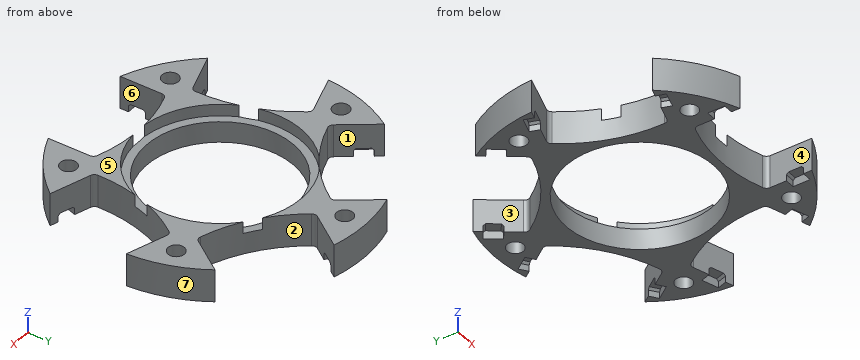
```python
from build123d import *

# Parameters (mm, degrees)
SKETCH1_R                = 28.194
SKETCH1_R_2              = 15.875
SKETCH1_R_3              = 14.2875
BOSS_EXTRUDE1_DEPTH      = 6.35
SKETCH1_3_R              = 15.875
SKETCH1_3_R_2            = 14.2875
CUT_EXTRUDE1_DEPTH       = 2.286
CUT_EXTRUDE5_DEPTH       = 7.35
CIRPATTERN1_COUNT        = 5
CUT_EXTRUDE6_DEPTH       = 1.8796
CIRPATTERN2_COUNT        = 5
CIRPATTERN2_COPY_1_DEPTH = 1.8796
CIRPATTERN2_COPY_2_DEPTH = 1.8796
CIRPATTERN2_COPY_3_DEPTH = 1.8796
CIRPATTERN2_COPY_4_DEPTH = 1.8796
SKETCH4_R                = 1.5875
CUT_EXTRUDE7_DEPTH       = 7.35
CIRPATTERN3_COUNT        = 5


with BuildPart() as part:
    # Sketch1 → Boss-Extrude1 (new body)
    with BuildSketch(Plane.XY):
        Circle(SKETCH1_R)
        Circle(SKETCH1_R_2, mode=Mode.SUBTRACT)
        Circle(SKETCH1_R_2)
        Circle(SKETCH1_R_3, mode=Mode.SUBTRACT)
    extrude(amount=-BOSS_EXTRUDE1_DEPTH)

    # Sketch1_3 → Cut-Extrude1 (cut)
    with BuildSketch(Plane.XY):
        Circle(SKETCH1_3_R)
        Circle(SKETCH1_3_R_2, mode=Mode.SUBTRACT)
    extrude(amount=-CUT_EXTRUDE1_DEPTH, mode=Mode.SUBTRACT)

    # Sketch2 → Cut-Extrude5 (cut, through all)
    with BuildSketch(Plane.XY):
        with BuildLine():
            Line((-10.033, -28.194), (10.033, -28.194))
            Line((10.033, -28.194), (10.033, -18.273516145))
            ThreePointArc((10.033, -18.273516145), (9.84417878, -17.683574397), (9.347899083, -17.312911233))
            ThreePointArc((9.347899083, -17.312911233), (0, -15.748), (-9.347899083, -17.312911233))
            ThreePointArc((-9.347899083, -17.312911233), (-9.84417878, -17.683574397), (-10.033, -18.273516145))
            Line((-10.033, -18.273516145), (-10.033, -28.194))
        make_face()
    cut_extrude5 = extrude(amount=-CUT_EXTRUDE5_DEPTH, mode=Mode.SUBTRACT)

    # CirPattern1: Cut-Extrude5 ×5 about axis
    cirpattern1_axis = Axis((0, 0, 0), (0, 0, 1))
    for i in range(1, CIRPATTERN1_COUNT):
        add(cut_extrude5.rotate(cirpattern1_axis, i * 360 / CIRPATTERN1_COUNT), mode=Mode.SUBTRACT)

    # Sketch3 → Cut-Extrude6 (cut)
    with BuildSketch(Plane(origin=(-10.033, 0, 0), x_dir=(0, 0, -1), z_dir=(1, 0, 0))):
        Polygon((6.35, -21.433544869), (5.15112, -21.433544869), (4.7498, -21.834864869), (4.7498, -24.334224869), (5.15112, -24.735544869), (6.35, -24.735544869), align=None)
    cut_extrude6 = extrude(amount=-CUT_EXTRUDE6_DEPTH, mode=Mode.SUBTRACT)

    # Mirror1: Cut-Extrude6 across plane
    add(cut_extrude6.mirror(Plane(origin=(0, 0, 0), x_dir=(0, 0, 1), z_dir=(1, 0, 0))), mode=Mode.SUBTRACT)

    # CirPattern2: Cut-Extrude6 ×5 about axis
    cirpattern2_axis = Axis((0, 0, 0), (0, 0, 1))
    for i in range(1, CIRPATTERN2_COUNT):
        add(cut_extrude6.rotate(cirpattern2_axis, i * 360 / CIRPATTERN2_COUNT), mode=Mode.SUBTRACT)

    # CirPattern2 copy 1 sketch → CirPattern2 copy 1 (cut)
    with BuildSketch(Plane(origin=(3.100367505, 9.541950028, 0), x_dir=(0, 0, -1), z_dir=(-0.309016994, -0.951056516, 0))):
        Polygon((6.35, 21.433544869), (5.15112, 21.433544869), (4.7498, 21.834864869), (4.7498, 24.334224869), (5.15112, 24.735544869), (6.35, 24.735544869), align=None)
    extrude(amount=-CIRPATTERN2_COPY_1_DEPTH, mode=Mode.SUBTRACT)

    # CirPattern2 copy 2 sketch → CirPattern2 copy 2 (cut)
    with BuildSketch(Plane(origin=(-8.116867505, 5.897249436, 0), x_dir=(0, 0, -1), z_dir=(0.809016994, -0.587785252, 0))):
        Polygon((6.35, 21.433544869), (5.15112, 21.433544869), (4.7498, 21.834864869), (4.7498, 24.334224869), (5.15112, 24.735544869), (6.35, 24.735544869), align=None)
    extrude(amount=-CIRPATTERN2_COPY_2_DEPTH, mode=Mode.SUBTRACT)

    # CirPattern2 copy 3 sketch → CirPattern2 copy 3 (cut)
    with BuildSketch(Plane(origin=(-8.116867505, -5.897249436, 0), x_dir=(0, 0, -1), z_dir=(0.809016994, 0.587785252, 0))):
        Polygon((6.35, 21.433544869), (5.15112, 21.433544869), (4.7498, 21.834864869), (4.7498, 24.334224869), (5.15112, 24.735544869), (6.35, 24.735544869), align=None)
    extrude(amount=-CIRPATTERN2_COPY_3_DEPTH, mode=Mode.SUBTRACT)

    # CirPattern2 copy 4 sketch → CirPattern2 copy 4 (cut)
    with BuildSketch(Plane(origin=(3.100367505, -9.541950028, 0), x_dir=(0, 0, -1), z_dir=(-0.309016994, 0.951056516, 0))):
        Polygon((6.35, 21.433544869), (5.15112, 21.433544869), (4.7498, 21.834864869), (4.7498, 24.334224869), (5.15112, 24.735544869), (6.35, 24.735544869), align=None)
    extrude(amount=-CIRPATTERN2_COPY_4_DEPTH, mode=Mode.SUBTRACT)

    # Sketch4 → Cut-Extrude7 (cut, through all)
    with BuildSketch(Plane(origin=(0, 0, -6.35), x_dir=(-1, 0, 0), z_dir=(0, 0, -1))):
        with Locations((-14.191068427, -19.532330016)):
            Circle(SKETCH4_R)
    cut_extrude7 = extrude(amount=-CUT_EXTRUDE7_DEPTH, mode=Mode.SUBTRACT)

    # CirPattern3: Cut-Extrude7 ×5 about axis
    cirpattern3_axis = Axis((0, 0, 0), (0, 0, 1))
    for i in range(1, CIRPATTERN3_COUNT):
        add(cut_extrude7.rotate(cirpattern3_axis, i * 360 / CIRPATTERN3_COUNT), mode=Mode.SUBTRACT)


solid = part.part
```
CAD build for the part. Positions are in the model's coordinates, mm. Face numbers are marked on the shaded views. A direction names the side the tool comes from. Round coordinates to 2 decimals unless told otherwise and drop trailing zeros. Loops run counter-clockwise (first coordinate to the right, second up) from the corner with the lowest first, then second, coordinate; pieces in that order, holes last. Notation, with made-up numbers: M 40.25,65.5 L 57.25,65.5 A30 cw 57.25,99.5 Z; hole C 2.25,13 d11. An arc over 180 degrees is marked long. Return JSON: item names as keys, results as strings. Group by question number.
(1) Wall check: probe 1 along Y at (x, z) = (0, -5); probe 2 along X at (y, z) = (12.5, -3.5). Give the ranges that are in metal, low to high. Write a range as [from, to].
(2) Drop flat-ended pins along their axis: P1, Ø2.5, axis at x = -14.19, y = -19.53, coming from the +Z side; P2, Ø2, axis at x = -25.5, y = 2.5, coming from the -Z side (3 decimals); P3, Ø1.3, axis at x = 18.5, y = -17.5, coming from the -Z side; P4, Ø1, axis at x = -11, z = -5.5, coming from the -Y side. Give the stop position or say it passes through.
(3) Saw through at A-A, the plane x = 0. Give the number of separate pieces and of enclosed holes in the cut face, and give its area (3 significant figures).
(4) Tool access for the marked faces 1, 2, 3 and 4: list every direction of +Z, -Z, +X, -X, +Y, -Y with a clear straight run to the whole face (end or side of a thin tool).
(5) Saw through at B-B, the plane y = -9. List the corners of the cut face in (x, z).
(6) Mould opens along X. For the marked faces 5, 6 and 7 say: +X half, -X half, draft (parallel to the pull), parting line (faces both ways), or undercut.
Answer list:
{
 "1": {"probe 1": "[-15.75, -14.29], [14.29, 22.56], [25.73, 28.19]", "probe 2": "[-25.27, -21.48], [-9.59, -6.92], [6.92, 9.59], [21.48, 25.27]"},
 "2": {"P1": "through", "P2": "z = -4.895", "P3": "z = -4.75", "P4": "y = -26.17"},
 "3": {"separate pieces": "3", "enclosed holes": "0", "area": "70.5 mm2"},
 "4": {"face 1": "+Z, -Z, +Y", "face 2": "+Z, -Z", "face 3": "+Z, -Z, -X", "face 4": "+Z, -Z, -Y"},
 "5": {"outline": "M -13.97,-6.35 L -11.1,-6.35 L -11.1,-2.29 L -13.08,-2.29 L -13.08,0 L -13.97,0 Z; M 11.1,-6.35 L 13.97,-6.35 L 13.97,0 L 13.08,0 L 13.08,-2.29 L 11.1,-2.29 Z"},
 "6": {"face 5": "draft", "face 6": "undercut", "face 7": "+X half"}
}
